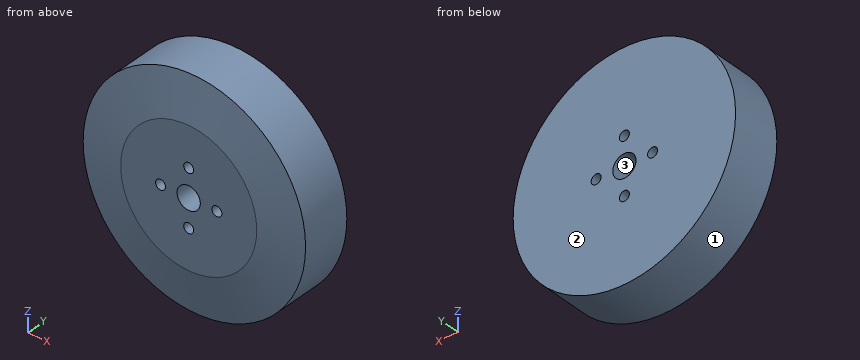
from build123d import *

# Parameters (mm, degrees)
SKETCH1_R               = 33.5
BOSS_EXTRUDE1_DEPTH     = 17
SKETCH2_R               = 3.5
CUT_EXTRUDE1_DEPTH      = 100
CUT_EXTRUDE1_DEPTH_BACK = 100
SKETCH3_R               = 1.5
CUT_EXTRUDE2_DEPTH      = 100
CUT_EXTRUDE2_DEPTH_BACK = 100
CHAMFER1_SIZE           = 13
CHAMFER1_SIZE2          = 2.058997724


with BuildPart() as part:
    # Sketch1 → Boss-Extrude1 (new body)
    with BuildSketch(Plane(origin=(0, 0, 0), x_dir=(1, 0, 0), z_dir=(0, 1, 0))):
        Circle(SKETCH1_R)
    extrude(amount=BOSS_EXTRUDE1_DEPTH)

    # Sketch2 → Cut-Extrude1 (cut, two sides)
    with BuildSketch(Plane(origin=(0, 0, 0), x_dir=(1, 0, 0), z_dir=(0, 1, 0))) as cut_extrude1_sk:
        Circle(SKETCH2_R)
    extrude(amount=CUT_EXTRUDE1_DEPTH, mode=Mode.SUBTRACT)
    extrude(cut_extrude1_sk.sketch, amount=-CUT_EXTRUDE1_DEPTH_BACK, mode=Mode.SUBTRACT)

    # Sketch3 → Cut-Extrude2 (cut, two sides)
    with BuildSketch(Plane(origin=(0, 0, 0), x_dir=(1, 0, 0), z_dir=(0, 1, 0))) as cut_extrude2_sk:
        with Locations((8.5, 0)):
            Circle(SKETCH3_R)
        with Locations((-8.5, 0)):
            Circle(SKETCH3_R)
        with Locations((0, -8.5)):
            Circle(SKETCH3_R)
        with Locations((0, 8.5)):
            Circle(SKETCH3_R)
    extrude(amount=CUT_EXTRUDE2_DEPTH, mode=Mode.SUBTRACT)
    extrude(cut_extrude2_sk.sketch, amount=-CUT_EXTRUDE2_DEPTH_BACK, mode=Mode.SUBTRACT)

    # Chamfer1
    chamfer1_edges = [part.edges().sort_by_distance(p)[0] for p in [
        (-33.5, 0, 0),
    ]]
    chamfer1_side = [part.faces().sort_by_distance(p)[0] for p in [
        (-32.552476913, 0, 0),
    ]]
    chamfer(chamfer1_edges, length=CHAMFER1_SIZE, length2=CHAMFER1_SIZE2, reference=chamfer1_side[0])


solid = part.part
CAD build for the part. Positions are in the model's coordinates, mm. Face numbers are marked on the shaded views. Coordinates: 2 decimals unless noted, no trailing zeros. Loops run counter-clockwise (first coordinate to the right, second up) from the corner with the lowest first, then second, coordinate; pieces in that order, holes last. Notation, with made-up numbers: (-0.75, 7.5) - (54.25, 7.5) arc R15 ccw to (54.25, 21.5) - close; hole circle Ø6 at (73, -34). An arc over 180 degrees is marked (long way). Write item = value, one per line. Start each with the question number.
Q1. Cut at A-A, the plane x = 0. List the corners of the cut face in (y, z).
Q2. Cut at B-B, the plane y = 14.25. List the corners of the cut face in (x, z).
Q3. Drill centre lines: L1, parallel to X at y = 12, z = 0; L2, parallel to X at y = 6.5, z = -8.5. Where is each one in solid material? Low to high.
Q4. Pull direction Z, two halves, no side cores. Call the marked faces 1, 2 and 3: pulls with the +Z half, pulls with the -Z half, needs draft (parallel to the pull), parting line crosses it, or undercut.
Q5. Flat gauge pins, fed straight in: pin 1 Ø10 at (y, z) = (7.5, -8) entering from -X; pin 2 Ø3.5 at (x, z) = (-8.5, 0) entering from -Y; pin 3 Ø4 at (y, z) = (12.5, -8.5) entering from +X; pin 4 Ø2.5 at (x, z) = (0, -8.5) entering from -Y. Where does each tip first touch, or does it go through?
Computed:
q1.outline = (0, -20.5) - (2.06, -33.5) - (17, -33.5) - (17, -10) - (0, -10) - close; (0, -7) - (17, -7) - (17, -3.5) - (0, -3.5) - close; (0, 3.5) - (17, 3.5) - (17, 7) - (0, 7) - close; (0, 10) - (17, 10) - (17, 33.5) - (2.06, 33.5) - (0, 20.5) - close
q2.outline = circle Ø67 at (0, 0); hole circle Ø3 at (-8.5, 0); hole circle Ø7 at (0, 0); hole circle Ø3 at (0, -8.5); hole circle Ø3 at (0, 8.5); hole circle Ø3 at (8.5, 0)
q3.L1 = -33.5 to -10, -7 to -3.5, 3.5 to 7, 10 to 33.5
q3.L2 = -32.4 to -1.5, 1.5 to 32.4
q4.face_1 = parting line crosses it
q4.face_2 = needs draft
q4.face_3 = undercut
q5.pin_1 = -33.37
q5.pin_2 = 0
q5.pin_3 = 32.86
q5.pin_4 = through
